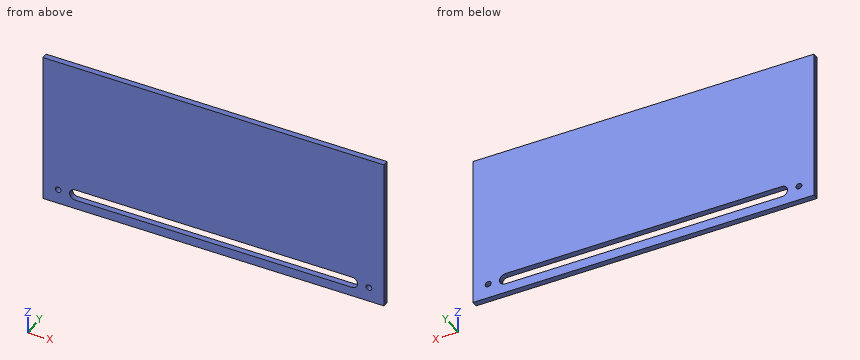
from build123d import *

# Parameters (mm, degrees)
F0_W     = 180
F0_H     = 83
F1_DEPTH = 3
F2_R     = 1.55
F2_W     = 152
F2_H     = 6
F3_DEPTH = 25
F4_R     = 2.99999


# Not quite as in the source:
# - a fillet or chamfer is up to 0.001 mm smaller than in the source, because OpenCascade refuses the exact size


with BuildPart() as f1:
    # F0 (on Front) → F1 (new body)
    with BuildSketch(Plane.XZ):
        with Locations((98.9931351204, 58.851495102)):
            Rectangle(F0_W, F0_H)
    extrude(amount=F1_DEPTH)

    # F2 (on face) → F3 (cut)
    with BuildSketch(Plane.XZ.offset(3)):
        with Locations((180.9931351204, 25.351495102)):
            Circle(F2_R)
        with Locations((98.9931351204, 25.351495102)):
            Rectangle(F2_W, F2_H)
        with Locations((16.9931351204, 25.351495102)):
            Circle(F2_R)
    extrude(amount=-F3_DEPTH, mode=Mode.SUBTRACT)

    # F4 (radius 3 in the source; OpenCascade refuses exactly that, so slightly less here)
    f4_edges = [f1.edges().sort_by_distance(p)[0] for p in [
        (22.993135, -1.5, 28.351495),
        (22.993135, -1.5, 22.351495),
        (174.993135, -1.5, 28.351495),
        (174.993135, -1.5, 22.351495),
    ]]
    fillet(f4_edges, radius=F4_R)


solid = f1.part
Work out the finished part from the listing and answer in its coordinate system (mm). Give positions to 0.01 mm unless a question says otherwise; leave off trailing zeros. Loops run counter-clockwise (first coordinate to the right, second up) from the corner with the lowest first, then second, coordinate; pieces in that order, holes last. Notation, with made-up numbers: (60.5, 87) - (84.5, 87) arc R17 ccw to (84.5, 117) - close; hole circle Ø10 at (-19.5, -28). An arc over 180 degrees is marked (long way). Answer in a Markdown table with one row per item.
(1) Consider L1, parallel to Z at x = 80, y = -2.3; L2, parallel to X at y = -1.85, z = 25. Determine where each line is inside the solid, lowest interval first. Write a range as [from, to].
Results list:
| item | result |
|---|---|
| L1 | z = [17.35, 22.35], [28.35, 100.35] |
| L2 | x = [8.99, 15.48], [18.5, 23.01], [174.97, 179.48], [182.5, 188.99] |
(2) Section A-A (x = 114) is taken. Give the vertices of the cut face in (y, z), and give its area (3 significant figures).
Results list:
| item | result |
|---|---|
| outline | (-3, 17.35) - (0, 17.35) - (0, 22.35) - (-3, 22.35) - close; (-3, 28.35) - (0, 28.35) - (0, 100.35) - (-3, 100.35) - close |
| area | 231 mm² |
(3) Section B-B (y = -0.6) is taken. State how many separate pieces and enclosed holes the cut face has, and give its area (3 significant figures).
Results list:
| item | result |
|---|---|
| separate pieces | 1 |
| enclosed holes | 3 |
| area | 14,000 mm² |
